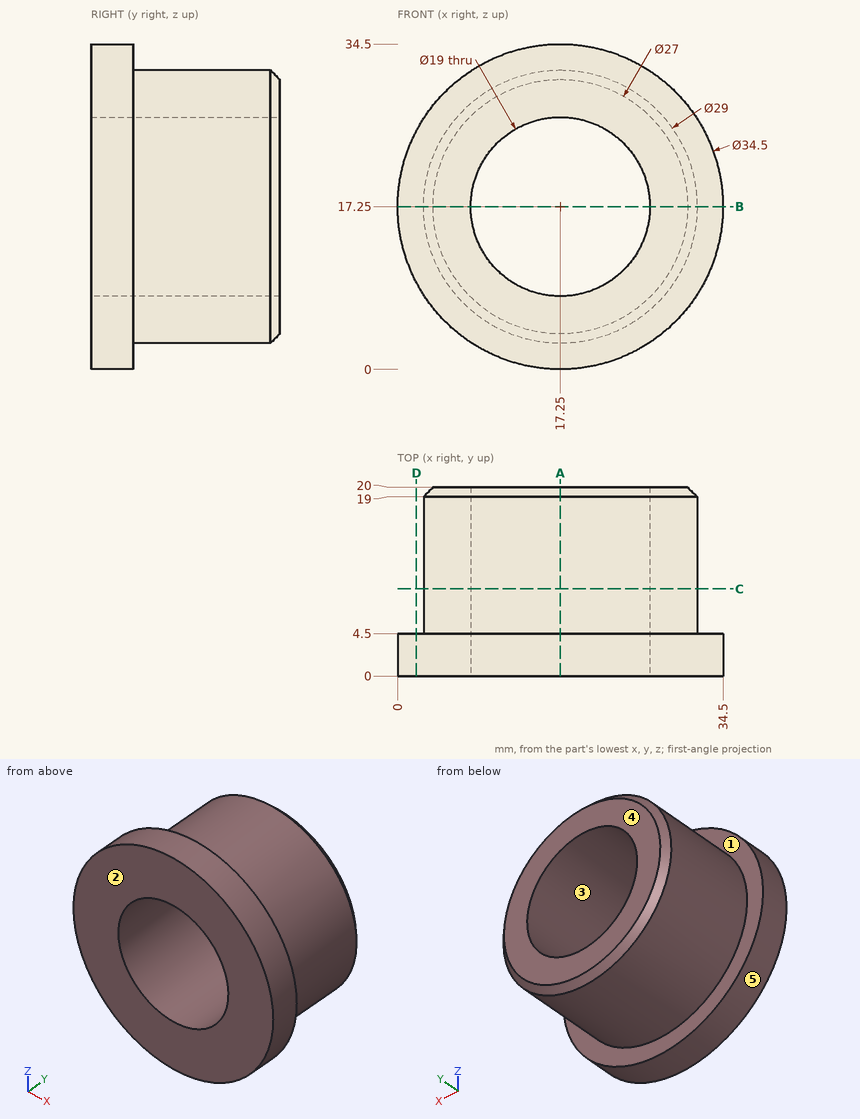
Can you work these out from the drawing? Everything is in mm from the part's minimum corner. A direction names the side the tool comes from. Give positions to 0.01 mm unless a question says otherwise; leave off trailing zeros. Loops run counter-clockwise (first coordinate to the right, second up) from the corner with the lowest first, then second, coordinate; pieces in that order, holes last. Notation, with made-up numbers: (72.5, -17.75) - (124.5, -17.75) arc R12 cw to (124.5, -8.75) - close; hole circle Ø5 at (-14.5, 17.5). An arc over 180 degrees is marked (long way). Answer as a JSON object with one key per item and string values.
Q1. Will these pins go through, and if not, where does the flat tip stop? P1, Ø3, axis at y = 17, z = 11.5, coming from the +X side; P2, Ø2, axis at x = 3.5, z = 29, coming from the +Y side; P3, Ø1.5, axis at x = 22, y = 15.5, coming from the -Z side.
Geometry says:
{"P1": "x = 31.11", "P2": "y = 4.5", "P3": "z = 3.31"}
Q2. Imagine slicing it at A-A on x = 17.25. Write out the boundary of the cut face in (y, z).
Geometry says:
{"outline": "(0, 0) - (4.5, 0) - (4.5, 2.75) - (19, 2.75) - (20, 3.75) - (20, 7.75) - (0, 7.75) - close; (0, 26.75) - (20, 26.75) - (20, 30.75) - (19, 31.75) - (4.5, 31.75) - (4.5, 34.5) - (0, 34.5) - close"}
Q3. Imagine slicing it at D-D on x = 2. Write out the boundary of the cut face in (y, z).
Geometry says:
{"outline": "(0, 9.19) - (4.5, 9.19) - (4.5, 25.31) - (0, 25.31) - close"}
Q4. Imagine slicing it at C-C on y = 9.25. Write out the boundary of the cut face in (x, z).
Geometry says:
{"outline": "circle Ø29 at (17.25, 17.25); hole circle Ø19 at (17.25, 17.25)"}
Q5. If we mould it in two halves opening along Z, with no side actions, what happens to the marked faces 3, 4 and 5? For each: pulls with the +Z half, pulls with the -Z half, needs draft (parallel to the pull), parting line crosses it, or undercut.
Geometry says:
{"face 3": "undercut", "face 4": "needs draft", "face 5": "parting line crosses it"}
Q6. Imagine slicing it at B-B on z = 17.25. Write out the boundary of the cut face in (x, y).
Geometry says:
{"outline": "(0, 0) - (7.75, 0) - (7.75, 20) - (3.75, 20) - (2.75, 19) - (2.75, 4.5) - (0, 4.5) - close; (26.75, 0) - (34.5, 0) - (34.5, 4.5) - (31.75, 4.5) - (31.75, 19) - (30.75, 20) - (26.75, 20) - close"}
Q7. Which directions (+Z, -Z, +X, -X, +Y, -Y) give clear straight access to the entire face, cutting with the end or side of a thin tool? Please do the marked faces 1 and 2.
Geometry says:
{"face 1": "+Y", "face 2": "+Z, -Z, +X, -X, -Y"}
Q8. If I drill on L1, parallel to X at y = 15, z = 17.25; L2, parallel to Z at x = 18.5, y = 10; L3, parallel to Y at x = 4.5, z = 6.5, over which ranges is the centre line in solid material (lowest first)?
Geometry says:
{"L1": "2.75 to 7.75, 26.75 to 31.75", "L2": "2.8 to 7.83, 26.67 to 31.7", "L3": "0 to 4.5"}
